```python
from build123d import *

# Parameters (mm, degrees)
BOSS_EXTRUDE_EQUERRE_DEPTH                     = 20
FRAISAGE_POUR_VIS_T_TE_FRAIS_E_M21_D           = 2.6
FRAISAGE_POUR_VIS_T_TE_FRAIS_E_M21_CSINK_D     = 4.4
FRAISAGE_POUR_VIS_T_TE_FRAIS_E_M21_CSINK_ANGLE = 90
TROU_TARAUD_M3X0_51_D                          = 2.5
TROU_TARAUD_M3X0_51_DEPTH                      = 10
TROU_TARAUD_M3X0_51_TIP                        = 0.751075774


with BuildPart() as part:
    # Esquisse1 → Boss_Extrude_Equerre (new body)
    with BuildSketch(Plane(origin=(0, 0, 0), x_dir=(0, 1, 0), z_dir=(0, 0, 1))):
        Polygon((0, 0), (32, 0), (32, 5), (-5, 5), (-5, 0), (-5, -27), (0, -27), align=None)
    extrude(amount=BOSS_EXTRUDE_EQUERRE_DEPTH)

    # Fraisage pour vis à tête fraisée M21 (through all)
    with Locations(Plane.ZY.offset(5)):
        with Locations((15, 29.5), (5, 29.5)):
            CounterSinkHole(FRAISAGE_POUR_VIS_T_TE_FRAIS_E_M21_D / 2, FRAISAGE_POUR_VIS_T_TE_FRAIS_E_M21_CSINK_D / 2, counter_sink_angle=FRAISAGE_POUR_VIS_T_TE_FRAIS_E_M21_CSINK_ANGLE)

    # Trou taraudé M3x0.51
    with Locations(Plane.YZ.offset(27)):
        with Locations((-2.5, 15), (-2.5, 5)):
            Hole(TROU_TARAUD_M3X0_51_D / 2, depth=TROU_TARAUD_M3X0_51_DEPTH)
            with Locations((0, 0, -(TROU_TARAUD_M3X0_51_DEPTH + TROU_TARAUD_M3X0_51_TIP / 2))):  # 118° drill point
                Cone(0, TROU_TARAUD_M3X0_51_D / 2, TROU_TARAUD_M3X0_51_TIP, mode=Mode.SUBTRACT)


solid = part.part
```
Geometry check sheet. Reference: the model listing, model coordinates, mm. A direction names the side the tool comes from. Coordinates: 2 decimals unless noted, no trailing zeros. Order: outer loops, then holes, each group sorted by start corner. A loop starts at its lowest first (then second) coordinate and runs counter-clockwise, first axis right, second up.
Item 1: Section check C-C (x = 1.5). Enter the section's corners in (y, z), plus the area to 3 significant figures.
Item 2: Depth check by flat-ended pin: pin 1 (6 mm diameter, centred on y = 20.5, z = 10, fed in from +X); pin 2 (10 mm diameter, centred on x = 15, z = 9.5, fed in from +Y). Enter the tip coordinate at first touch or a pass-through.
Item 3: Tool access check on faces 1 (the cylindrical face through (-2.02, 29.56, 16.3)), 2 (the flat face through (14, 0, 10)). Record the directions out of +Z, -Z, +X, -X, +Y, -Y that give a thin tool (end or side, any length) a straight path to the whole face; none if there is none.
Item 4: Mould release check, pull along Y, two halves, no side actions. Record for faces 3 (the cylindrical face through (21.93, -3.077, 3.891)), 4 (the cylindrical face through (21.93, -3.172, 16.054)), 5 (the flat face through (-2, 32, 10)), 6 (the flat face through (0, 16, 10)): released by +Y, released by -Y, zero draft, split by the parting line, or undercut.
Item 5: Scan lines: line 1 along Z through (x, y) = (22.75, -2.5); line 2 along Z through (x, y) = (-2.7, 29.5); line 3 along Y through (x, z) = (-1.7, 15). Record each from-to range of solid material in increasing order.
Item 6: Section check B-B (z = 18). Enter the section's corners in (x, y), plus the area to 3 significant figures.
Item 7: Section check A-A (y = 29.5). Enter the section's corners in (x, z), plus the area to 3 significant figures.
Check sheet entries:
1. outline: (-5, 0) - (0, 0) - (0, 20) - (-5, 20) - close
1. area: 100 mm2
2. pin 1: stops at x = 0
2. pin 2: stops at y = 0
3. face 1: +X, -X
3. face 2: +Z, -Z, +X, +Y
4. face 3: undercut
4. face 4: undercut
4. face 5: released by +Y
4. face 6: zero draft
5. line 1: z = 0 to 3.75, 6.25 to 13.75, 16.25 to 20
5. line 2: z = 0 to 3.7, 6.3 to 13.7, 16.3 to 20
5. line 3: y = -5 to 28.2, 30.8 to 32
6. outline: (-5, -5) - (27, -5) - (27, 0) - (0, 0) - (0, 32) - (-5, 32) - close
6. area: 320 mm2
7. outline: (-5, 0) - (0, 0) - (0, 3.7) - (-4.1, 3.7) - (-5, 2.8) - close; (-5, 7.2) - (-4.1, 6.3) - (0, 6.3) - (0, 13.7) - (-4.1, 13.7) - (-5, 12.8) - close; (-5, 17.2) - (-4.1, 16.3) - (0, 16.3) - (0, 20) - (-5, 20) - close
7. area: 72.4 mm2
